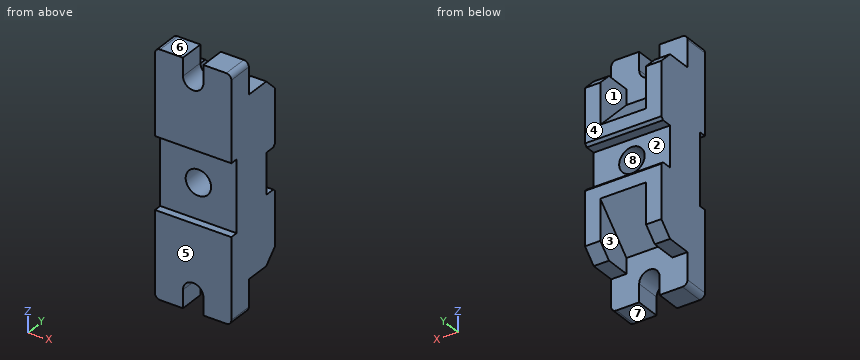
Autodesk Inventor part; units mm, degrees
ref_plane "YZ Plane" through (0, 0, 0) normal (1, 0, 0) x (0, 1, 0)
ref_plane "XZ Plane" through (0, 0, 0) normal (0, 1, 0) x (-1, 0, 0)
ref_plane "XY Plane" through (0, 0, 0) normal (0, 0, 1) x (1, 0, 0)
sketch "Schizzo1" plane through (0, 0, 0) normal (0, 1, 0) x (-1, 0, 0)
  line L0 (0, 0) -> (15, 0) construction
  line L1 (15, 0) -> (15, -47.5)
  line L2 (15, -47.5) -> (4, -47.5)
  line L3 (4, -47.5) -> (4, -40.5)
  line L4 (0, 0) -> (0, -36.5) construction
  arc A0 (4, -40.5) -> (0, -36.5) centre (0, -40.5) ccw
  arc A1 (0, -5) -> (5, 0) centre (0, 0) ccw
  line L5 (0, 0) -> (0, -8) construction
  line L6 (0, -8) -> (15, -8)
  line L7 (15, 0) -> (15, -14)
  line L8 (15, -14) -> (0, -14)
  line L9 (15, -35) -> (9, -35)
  line L10 (9, -35) -> (9, -14)
  line L11 (0, 0) -> (-15, 0) construction
  line L12 (-15, 0) -> (-15, -47.5)
  line L13 (-15, -47.5) -> (-4, -47.5)
  line L14 (-4, -47.5) -> (-4, -40.5)
  arc A2 (0, -36.5) -> (-4, -40.5) centre (0, -40.5) ccw
  arc A3 (-5, 0) -> (0, -5) centre (0, 0) ccw
  line L15 (0, -8) -> (-15, -8)
  line L16 (-15, 0) -> (-15, -14)
  line L17 (-15, -14) -> (0, -14)
  line L18 (-15, -35) -> (-9, -35)
  line L19 (-9, -35) -> (-9, -14)
  line L20 (15, 0) -> (15, 47.5)
  line L21 (15, 47.5) -> (4, 47.5)
  line L22 (4, 47.5) -> (4, 40.5)
  line L23 (0, 0) -> (0, 36.5) construction
  arc A4 (0, 36.5) -> (4, 40.5) centre (0, 40.5) ccw
  arc A5 (5, 0) -> (0, 5) centre (0, 0) ccw
  line L24 (0, 0) -> (0, 8) construction
  line L25 (0, 8) -> (15, 8)
  line L26 (15, 0) -> (15, 14)
  line L27 (15, 14) -> (0, 14)
  line L28 (15, 35) -> (9, 35)
  line L29 (9, 35) -> (9, 14)
  arc A6 (-4, 40.5) -> (0, 36.5) centre (0, 40.5) ccw
  line L30 (-15, 47.5) -> (-4, 47.5)
  line L31 (-4, 47.5) -> (-4, 40.5)
  line L32 (-15, 35) -> (-9, 35)
  line L33 (-15, 14) -> (0, 14)
  line L34 (-9, 35) -> (-9, 14)
  line L35 (-15, 0) -> (-15, 47.5)
  line L36 (0, 8) -> (-15, 8)
  arc A7 (0, 5) -> (-5, 0) centre (0, 0) ccw
  line L37 (-15, 0) -> (-15, 14)
  dimension "d0" = 15
  dimension "d1" = 47.5
  dimension "d2" = 11
  dimension "d5" = 5
  dimension "d6" = 8
  dimension "d7" = 14
  dimension "d8" = 6
extrude "Estrusione1" add sketch "Schizzo1" along normal blind 10 contours L1 L2 L3 A0 A2 L14 L13 L12 L18 L19 L17 L8 L10 L9 | L28 L29 L27 L33 L34 L32 L35 L30 L31 A6 A4 L22 L21 L20
extrude "Estrusione2" add sketch "Schizzo1" along normal blind 25 contours L1 L8 L17 L12 L15 L6 | L25 L36 L35 L33 L27 L20 | L1 L9 L10 L8 | L27 L29 L28 L20 | L17 L19 L18 L12 | L35 L32 L34 L33
extrude "Estrusione3" add sketch "Schizzo1" along normal blind 20 contours L1 L6 L15 L12 L35 L36 L25 L20
sketch "Schizzo1 outline for Estrusione4" plane through (0, 0, 0) normal (0, 1, 0) x (-1, 0, 0)
  line L0 (-15, 0) -> (-15, -14)
  line L1 (-15, 14) -> (-15, 0)
  line L2 (-15, -14) -> (0, -14)
  line L3 (0, 14) -> (-15, 14)
  line L4 (0, -14) -> (15, -14)
  line L5 (15, 14) -> (0, 14)
  line L6 (15, -14) -> (15, 0)
  line L7 (15, 0) -> (15, 14)
  arc A0 (0, -5) -> (-5, 0) centre (0, 0) cw
  arc A1 (5, 0) -> (0, -5) centre (0, 0) cw
  arc A2 (0, 5) -> (5, 0) centre (0, 0) cw
  arc A3 (-5, 0) -> (0, 5) centre (0, 0) cw
extrude "Estrusione4" cut sketch "Schizzo1 outline for Estrusione4" along normal blind 3
chamfer "Smusso1" distance 15 angle 45 1 edges at (0, 10, 14) measured on face at (-3, 15, 14)
chamfer "Smusso2" distance 15 angle 45 1 edges at (0, 10, -14) measured on face at (3, 15, -14)
chamfer "Smusso3" distance 5 angle 45 2 edges at (-12, 25, -35) (12, 25, -35) measured on face at (3, 25, -10)
chamfer "Smusso4" distance 5 angle 45 2 edges at (12, 25, 35) (-12, 25, 35) measured on face at (-3, 25, 10)
fillet "Raccordo1" radius 2 4 edges at (-15, 5, -47.5) (-15, 5, 47.5) (15, 5, 47.5) (15, 5, -47.5)
chamfer "Smusso5" distance 1 angle 45 1 edges at (0, 25, -8) measured on face at (-3, 25, -10)
chamfer "Smusso6" distance 1 angle 45 1 edges at (0, 25, 8) measured on face at (-3, 25, 10)
properties part number "esercizio 040.30 03-02-2023"
Geometry check sheet. Reference: the model listing, model coordinates, mm. Face numbers are marked on the shaded views. A direction names the side the tool comes from. Coordinates: 2 decimals unless noted, no trailing zeros. Order: outer loops, then holes, each group sorted by start corner. A loop starts at its lowest first (then second) coordinate and runs counter-clockwise, first axis right, second up. Notation, with made-up numbers: (8, 16.5) - (23, 16.5) arc R31 cw to (23, 51.5) - close; hole circle Ø2 at (-31, -37.75). An arc over 180 degrees is marked (long way). Answer in a Markdown table with one row per item. Add a question column.
1) Cross-section at D-D, the plane y = 2. Record the cut outline in (x, z), then the cut area to 3 significant figures.
2) Material ranges on line 1 along X through (y, z) = (9, 0); line 2 along Z through (x, y) = (0, 8.25); line 3 along Y through (x, z) = (-13.25, -5.5), recorded low to high. Write a range as [from, to].
3) Cross-section at A-A, the plane z = 0. Record the cut outline in (x, y), then the cut area to 3 significant figures.
4) Set-up check for the marked faces 1, 2, 3, 4 and 5: record each of +Z, -Z, +X, -X, +Y, -Y from which the full face is reachable in a straight line by a thin tool's end or side.
5) Cross-section at C-C, the plane y = 8.75. Record the cut outline in (x, z), then the cut area to 3 significant figures.
6) Release check for a two-part mould opening along Z. For the marked faces 6, 7 and 8 record: +Z half, -Z half, draft (parallel to the pull), parting line (faces both ways), or undercut.
7) Gauge pin test, flat ends, axial feed: P1, Ø15, axis at x = 3.5, z = 35, coming from the +Y side; P2, Ø4, axis at x = 2, z = 3, coming from the +Y side; P3, Ø5.5, axis at x = -4, z = -35.5, coming from the +Y side; P4, Ø1.8, axis at x = -12.5, y = 17, coming from the -Z side. Record the tip position at first contact, or that the pin passes through.
Check result:
| question | item | result |
|---|---|---|
| 1 | outline | (-15, -45.5) arc R2 ccw to (-13, -47.5) - (-4, -47.5) - (-4, -40.5) arc R4 cw to (4, -40.5) - (4, -47.5) - (13, -47.5) arc R2 ccw to (15, -45.5) - (15, -14) - (-15, -14) - close; (-15, 14) - (15, 14) - (15, 45.5) arc R2 ccw to (13, 47.5) - (4, 47.5) - (4, 40.5) arc R4 cw to (-4, 40.5) - (-4, 47.5) - (-13, 47.5) arc R2 ccw to (-15, 45.5) - close |
| 1 | area | 1,840 mm² |
| 2 | line 1 | x = [-15, -5], [5, 15] |
| 2 | line 2 | z = [-36.5, -5], [5, 36.5] |
| 2 | line 3 | y = [3, 20] |
| 3 | outline | (-15, 3) - (-5, 3) - (-5, 20) - (-15, 20) - close; (5, 3) - (15, 3) - (15, 20) - (5, 20) - close |
| 3 | area | 340 mm² |
| 4 | face 1 | +Z, +Y |
| 4 | face 2 | +X, -X, +Y |
| 4 | face 3 | -Z, +Y |
| 4 | face 4 | +Z, -Z, +X, -X, +Y |
| 4 | face 5 | +Z, -Z, +X, -X, -Y |
| 5 | outline | (-15, -45.5) arc R2 ccw to (-13, -47.5) - (-4, -47.5) - (-4, -40.5) arc R4 cw to (4, -40.5) - (4, -47.5) - (13, -47.5) arc R2 ccw to (15, -45.5) - (15, 45.5) arc R2 ccw to (13, 47.5) - (4, 47.5) - (4, 40.5) arc R4 cw to (-4, 40.5) - (-4, 47.5) - (-13, 47.5) arc R2 ccw to (-15, 45.5) - close; hole circle Ø10 at (0, 0) |
| 5 | area | 2,610 mm² |
| 6 | face 6 | +Z half |
| 6 | face 7 | -Z half |
| 6 | face 8 | undercut |
| 7 | P1 | stops at y = 25 |
| 7 | P2 | stops at y = 20 |
| 7 | P3 | stops at y = 10 |
| 7 | P4 | stops at z = -35 |
